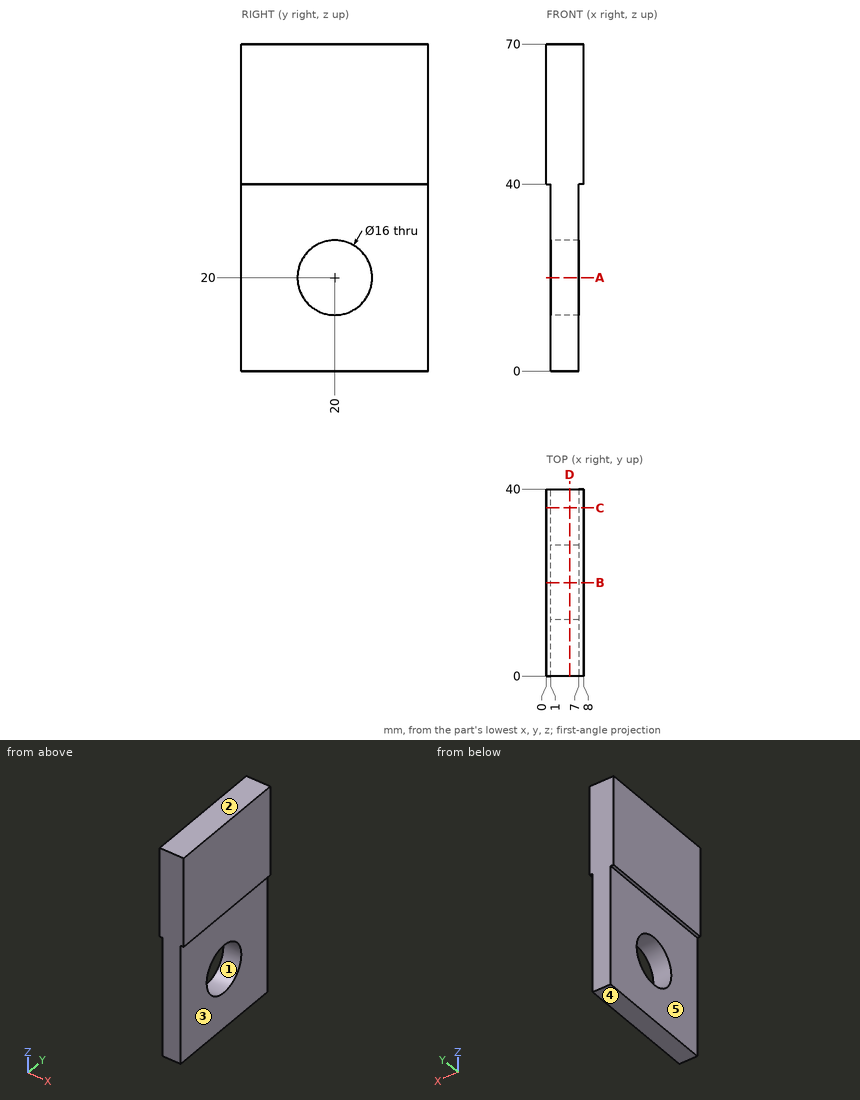
Study the drawing (mm; zero at the part's minimum x, y, z) and answer. A direction names the side the tool comes from. Round coordinates to 2 decimals unless told otherwise and drop trailing zeros. Loops run counter-clockwise (first coordinate to the right, second up) from the corner with the lowest first, then second, coordinate; pieces in that order, holes last. Notation, with made-up numbers: (5, 13) -> (57, 13) arc R11 cw to (57, 31) -> close; hole circle Ø9 at (50, -34.75). An arc over 180 degrees is marked (long way). Write each question's results on one line, items separated by ' | '. Start each with the question number.
1. Section D-D (x = 5) is taken. Determine the outline of the cut face in (y, z).
2. Section C-C (y = 36) is taken. Determine the outline of the cut face in (x, z).
3. Section B-B (y = 20) is taken. Determine the outline of the cut face in (x, z).
4. Find the intervals of material crossed by probe 1 along Y at (x, z) = (4.75, 20); probe 2 along X at (y, z) = (22, 30.5); probe 3 along Z at (x, y) = (6, 21), in increasing order. Write a range as from..to.
5. A tool of negligible diameter and unlimited length cuts with its end or side. For the marked faces 4 and 5, from which of +Z, -Z, +X, -X, +Y, -Y can it reach the whole face along a straight path? Write none if from no direction.
6. Section A-A (z = 20) is taken. Determine the outline of the cut face in (x, y).
7. For a pull along Z with two mould halves and no side action, classify the marked faces 1, 2 and 3 as +Z half, -Z half, draft (parallel to the pull), parting line (faces both ways), or undercut.
8. Given pin 1 Ø0.5 at (x, y) = (7.5, 17.5) entering from -Z; pin 2 Ø18.5 at (y, z) = (20, 20) entering from -X; pin 3 Ø1.5 at (y, z) = (14, 28.5) entering from +X; pin 4 Ø1.1 at (x, y) = (0.5, 17) entering from -Z, each flat-ended and moving along its own axis, determine where each tip first touches the part or whether it passes through.
Evaluation:
1) outline: (0, 0) -> (40, 0) -> (40, 70) -> (0, 70) -> close; hole circle Ø16 at (20, 20)
2) outline: (0, 40) -> (1, 40) -> (1, 0) -> (7, 0) -> (7, 40) -> (8, 40) -> (8, 70) -> (0, 70) -> close
3) outline: (0, 40) -> (1, 40) -> (1, 28) -> (7, 28) -> (7, 40) -> (8, 40) -> (8, 70) -> (0, 70) -> close; (1, 0) -> (7, 0) -> (7, 12) -> (1, 12) -> close
4) probe 1: y = 0..12, 28..40 | probe 2: x = 1..7 | probe 3: z = 0..12.06, 27.94..70
5) face 4: -Z, +X, -X, +Y, -Y | face 5: -Z, -X, +Y, -Y
6) outline: (1, 0) -> (7, 0) -> (7, 12) -> (1, 12) -> close; (1, 28) -> (7, 28) -> (7, 40) -> (1, 40) -> close
7) face 1: undercut | face 2: +Z half | face 3: draft
8) pin 1: stops at z = 40 | pin 2: stops at x = 1 | pin 3: stops at x = 7 | pin 4: stops at z = 0
